from build123d import *

# Parameters (mm, degrees)
SKETCH9_W                                       = 56.5
SKETCH9_H                                       = 39
BOSS_EXTRUDE7_DEPTH                             = 33.5
CUT_EXTRUDE3_DEPTH                              = 28.5
SKETCH12_W                                      = 36.5
SKETCH12_H                                      = 28.5
CUT_EXTRUDE4_DEPTH                              = 56.464515683
CBORE_FOR_M3_SOCKET_HEAD_CAP_SCREW3_D           = 3.2
CBORE_FOR_M3_SOCKET_HEAD_CAP_SCREW3_CBORE_D     = 6.5
CBORE_FOR_M3_SOCKET_HEAD_CAP_SCREW3_CBORE_DEPTH = 3
F_2_0MM_DOWEL_HOLE1_D                           = 2
F_2_0MM_DOWEL_HOLE1_CSINK_D                     = 2.05
F_2_0MM_DOWEL_HOLE1_CSINK_ANGLE                 = 90


with BuildPart() as part:
    # Sketch9 → Boss-Extrude7 (new body)
    with BuildSketch(Plane(origin=(0, 0, 0), x_dir=(1, 0, 0), z_dir=(0, 1, 0))):
        Rectangle(SKETCH9_W, SKETCH9_H)
    extrude(amount=BOSS_EXTRUDE7_DEPTH)

    # Sketch11 → Cut-Extrude3 (cut)
    with BuildSketch(Plane(origin=(0, 33.5, 0), x_dir=(1, 0, 0), z_dir=(0, 1, 0))):
        Polygon((-23.25, -14.5), (-23.25, -19.5), (23.25, -19.5), (23.25, -14.5), (23.25, 14.5), (-23.25, 14.5), align=None)
    extrude(amount=-CUT_EXTRUDE3_DEPTH, mode=Mode.SUBTRACT)

    # Sketch12 → Cut-Extrude4 (cut, through all)
    with BuildSketch(Plane.XY.offset(-14.5)):
        with Locations((0, 19.25)):
            Rectangle(SKETCH12_W, SKETCH12_H)
    extrude(amount=-CUT_EXTRUDE4_DEPTH, mode=Mode.SUBTRACT)

    # CBORE for M3 Socket Head Cap Screw3 (through all)
    with Locations(Plane(origin=(10, 5, -10), x_dir=(0, 0, 1), z_dir=(0, 1, 0))):
        with Locations((0, 0), (20, 0), (20, -20), (0, -20)):
            CounterBoreHole(CBORE_FOR_M3_SOCKET_HEAD_CAP_SCREW3_D / 2, CBORE_FOR_M3_SOCKET_HEAD_CAP_SCREW3_CBORE_D / 2, CBORE_FOR_M3_SOCKET_HEAD_CAP_SCREW3_CBORE_DEPTH)

    # Ø2.0mm Dowel Hole1 (through all)
    with Locations(Plane(origin=(28.25, 0, 0), x_dir=(0, 0, -1), z_dir=(1, 0, 0))):
        with Locations((-8.5, 27.5), (-8.5, 11.5), (3.5, 11.5), (3.5, 27.5)):
            CounterSinkHole(F_2_0MM_DOWEL_HOLE1_D / 2, F_2_0MM_DOWEL_HOLE1_CSINK_D / 2, counter_sink_angle=F_2_0MM_DOWEL_HOLE1_CSINK_ANGLE)


solid = part.part
Source: CAD feature listing. Evaluate the final solid. Frame: model axes, mm. A direction names the side the tool comes from. Round coordinates to 2 decimals unless told otherwise and drop trailing zeros. Loops run counter-clockwise (first coordinate to the right, second up) from the corner with the lowest first, then second, coordinate; pieces in that order, holes last. Notation, with made-up numbers: M 46,-34 L 62,-34 A28 cw 62,-16 Z; hole C -27,41 d9. An arc over 180 degrees is marked long. Answer as CSV lines item,"result".
Q1. Cut plane C-C (z = -3.5). Return the cut outline in (x, y) (3 decimals).
Verdict:
outline,"M -28.25,0 L 28.25,0 L 28.25,10.475 L 28.225,10.5 L 23.25,10.5 L 23.25,5 L -23.25,5 L -23.25,10.5 L -28.25,10.5 Z; M -28.25,12.5 L -23.25,12.5 L -23.25,26.5 L -28.25,26.5 Z; M -28.25,28.5 L -23.25,28.5 L -23.25,33.5 L -28.25,33.5 Z; M 23.25,12.5 L 28.225,12.5 L 28.25,12.525 L 28.25,26.475 L 28.225,26.5 L 23.25,26.5 Z; M 23.25,28.5 L 28.225,28.5 L 28.25,28.525 L 28.25,33.5 L 23.25,33.5 Z"
Q2. Contact query for flat-ended pins moving along their axis: pin 1 (2 mm diameter, centred on x = 9.5, z = 11, fed in from +Y); pin 2 (7 mm diameter, centred on x = -9, z = -11, fed in from +Y). Output: stop coordinate, or through.
Verdict:
pin 1,"stops at y = 2"
pin 2,"stops at y = 5"
Q3. Line query: line 1 along X through (y, z) = (1.35, 10); line 2 along Z through (x, y) = (26.2, 27.5); line 3 along X through (y, z) = (30, -9.5). Output: solid intervals per line, ascending.
Verdict:
line 1,"x = -28.25 to -11.6, -8.4 to 8.4, 11.6 to 28.25"
line 2,"z = -19.5 to -4.5, -2.5 to 7.5, 9.5 to 19.5"
line 3,"x = -28.25 to -23.25, 23.25 to 28.25"
Q4. Cut plane D-D (x = 10). Return the cut outline in (y, z), plus the area to 3 significant figures.
Verdict:
outline,"M 0,-19.5 L 5,-19.5 L 5,-13.25 L 2,-13.25 L 2,-11.6 L 0,-11.6 Z; M 0,-8.4 L 2,-8.4 L 2,-6.75 L 5,-6.75 L 5,6.75 L 2,6.75 L 2,8.4 L 0,8.4 Z; M 0,11.6 L 2,11.6 L 2,13.25 L 5,13.25 L 5,19.5 L 0,19.5 Z"
area,"143 mm^2"
Q5. Cut plane B-B (y = 27.5). Count the separate pieces of the cut face and the enclosed holes in it, plus the area to 3 significant figures.
Verdict:
separate pieces,"6"
enclosed holes,"0"
area,"400 mm^2"
Q6. Pull-direction query (X, two-part tool) for faces 4 (the face through (28.25, 17, 0)), 5 (the face through (0, 2, -19.5)), 6 (the face through (10.07, 0.99, 11.6)), 7 (the face through (-7.803, 3.521, 7.605)); classes: +X half, -X half, draft (parallel to the pull), parting line (faces both ways), or undercut.
Verdict:
face 4,"+X half"
face 5,"draft"
face 6,"undercut"
face 7,"undercut"
Q7. Reachability of faces 1 (the face through (21, 19, -14.5)), 2 (the face through (-11.4, 2, 11.4)), 3 (the face through (-25.78, 28.49, 8.37)) from +Z, -Z, +X, -X, +Y, -Y: full face, straight path, thin tool, end or side. Return the list, or none.
Verdict:
face 1,"+Z, +Y"
face 2,"+Y"
face 3,"+X, -X"
Q8. Cut plane A-A (z = -10). Return the cut outline in (x, y), plus the area to 3 significant figures.
Verdict:
outline,"M -28.25,0 L -11.6,0 L -11.6,2 L -13.25,2 L -13.25,5 L -23.25,5 L -23.25,33.5 L -28.25,33.5 Z; M -8.4,0 L 8.4,0 L 8.4,2 L 6.75,2 L 6.75,5 L -6.75,5 L -6.75,2 L -8.4,2 Z; M 11.6,0 L 28.25,0 L 28.25,33.5 L 23.25,33.5 L 23.25,5 L 13.25,5 L 13.25,2 L 11.6,2 Z"
area,"516 mm^2"
